Part print with two shaded views. Sizes in mm from the minimum x, y, z corner. Coordinates: 2 decimals unless noted, no trailing zeros. Write each loop counter-clockwise with the first axis right and the second up, starting at its lowest first coordinate (ties: lowest second). Pieces come first, ordered by that corner, then holes. Notation, with made-up numbers: (51.5, 4.25) - (56.5, 4.25) arc R31 cw to (56.5, 42.25) - close; hole circle Ø3 at (-8.5, 54.5). An arc over 180 degrees is marked (long way). Answer in a Markdown table with one row per item. Add a question column.
Q1. Pin check, flat tips, straight feed: pin 1 (4 mm diameter, centred on x = 29.5, z = 7, fed in from +Y); pin 2 (1 mm diameter, centred on y = 32, z = 3.5, fed in from -X); pin 3 (1.6 mm diameter, centred on y = 22.5, z = 7, fed in from -X); pin 4 (3.5 mm diameter, centred on y = 23, z = 7.5, fed in from +X) (3 decimals). Stop position of each tip, or through.
Q2. Band-saw the part on C-C (x = 13.5). List the corners of the cut face in (y, z) (3 decimals), and give its area (3 significant figures).
Q3. Drill centre lines: line 1 along Z through (x, y) = (13, 2.5) (3 decimals); line 2 along Y through (x, z) = (6.5, 3.75). Where is each one in solid material? Low to high. Write a range as from..to.
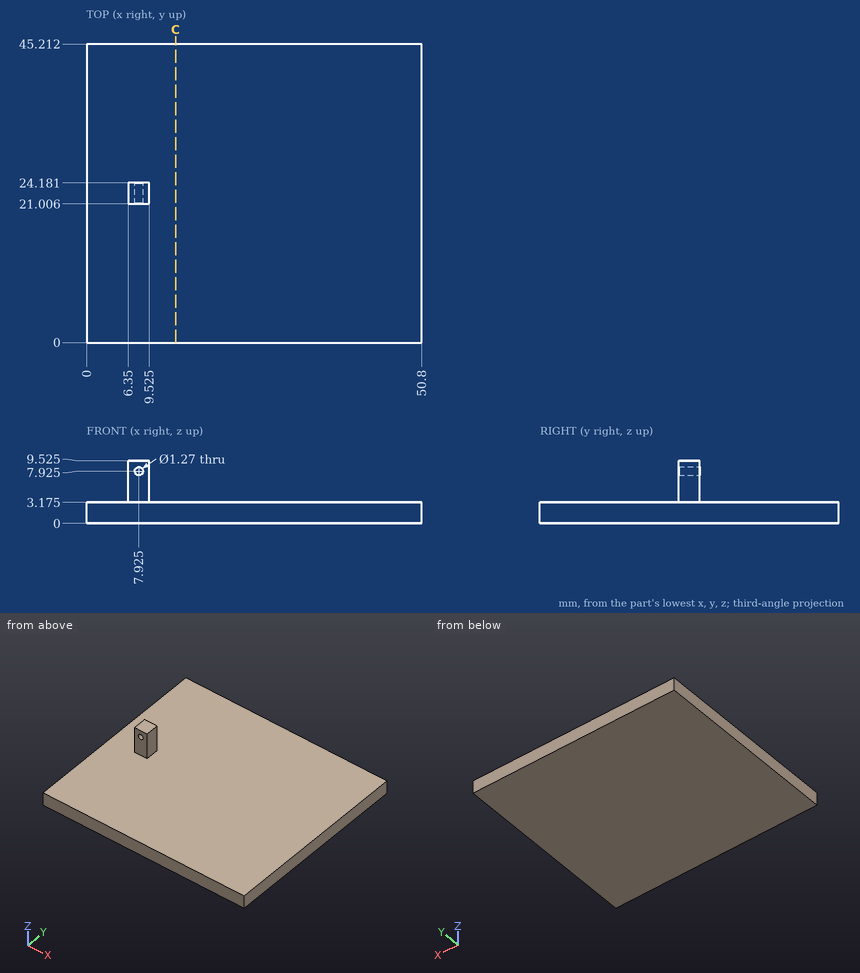
Checked values:
| question | item | result |
|---|---|---|
| 1 | pin 1 | passes through |
| 1 | pin 2 | stops at x = 0 |
| 1 | pin 3 | stops at x = 6.35 |
| 1 | pin 4 | stops at x = 9.525 |
| 2 | outline | (0, 0) - (45.212, 0) - (45.212, 3.175) - (0, 3.175) - close |
| 2 | area | 144 mm² |
| 3 | line 1 | z = 0..3.175 |
| 3 | line 2 | y = 21.01..24.18 |
